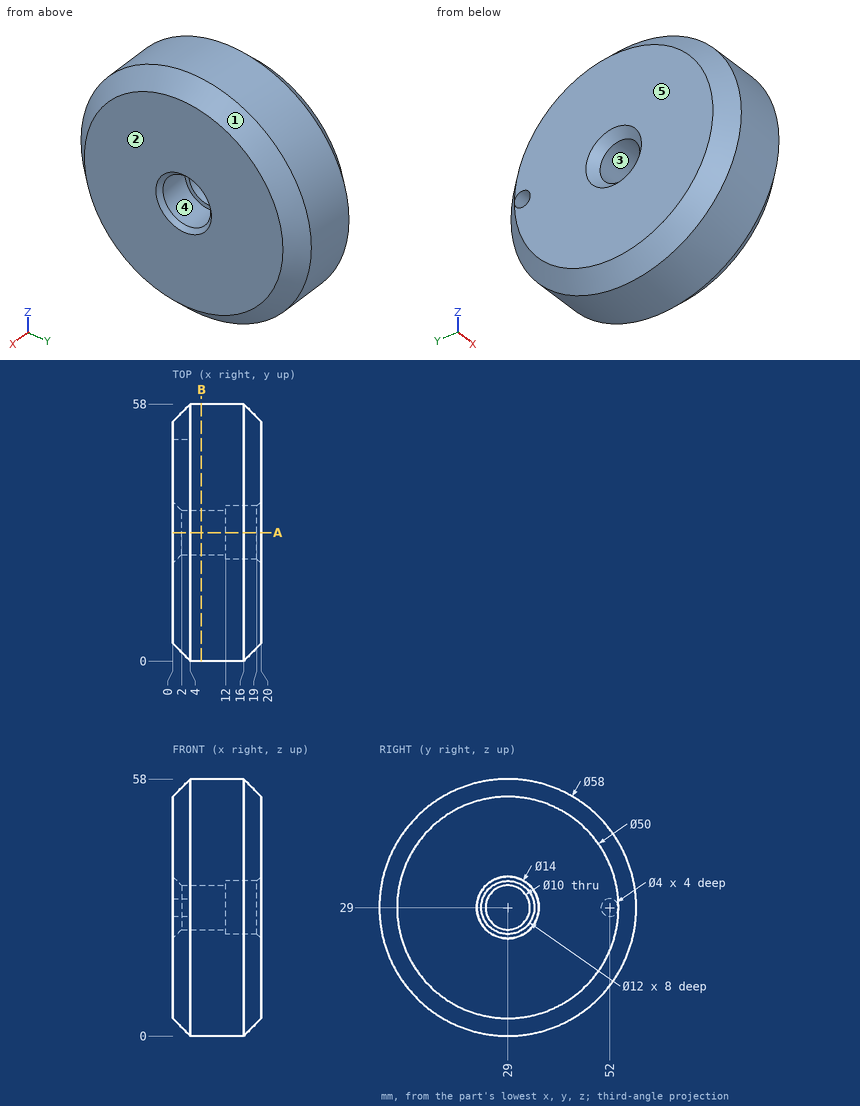
Drawing for the job (mm, zero at the part's lowest x, y, z). A direction names the side the tool comes from. Round coordinates to 2 decimals unless told otherwise and drop trailing zeros. Order: outer loops, then holes, each group sorted by start corner. A loop starts at its lowest first (then second) coordinate and runs counter-clockwise, first axis right, second up. Notation, with made-up numbers: (0, 12.25) -> (59, 12.25) arc R22 ccw to (59, 48.25) -> close; hole circle Ø10 at (-2.5, -12.75). An arc over 180 degrees is marked (long way). Write item = value, one per line. Start each with the question number.
(1) Pin check, flat tips, straight feed: P1, Ø2, axis at x = 9.5, z = 18, coming from the +Y side; P2, Ø8, axis at x = 14, y = 16.5, coming from the +Z side; P3, Ø1.5, axis at x = 12.5, z = 8.5, coming from the +Y side. Stop position of each tip, or through.
(2) Cut at A-A, the plane y = 29. List the corners of the cut face in (x, z).
(3) Probe line 1 (Z direction, x = 14.5, y = 29); line 2 (Z direction, x = 6, y = 29); line 3 (Y direction, x = 17.75, z = 29). List the from-to ranges inside material, lowest first. Write a range as [from, to].
(4) Pull direction Y, two halves, no side cores. Call the marked faces 1, 2 and 3: released by +Y, released by -Y, zero draft, split by the parting line, or undercut.
(5) Cut at B-B, the plane x = 6.5. List the corners of the cut face in (y, z).
(6) Which spindle directions (+Z, -Z, +X, -X, +Y, -Y) get a long thin tool onto all of the face, cutting with end or side? Do the marked faces 4 and 5. Say none if no direction does.
Model answer:
q1.P1 = 56.22
q1.P2 = 56.73
q1.P3 = 50.24
q2.outline = (0, 4) -> (4, 0) -> (16, 0) -> (20, 4) -> (20, 22) -> (19, 23) -> (12, 23) -> (12, 24) -> (2, 24) -> (0, 22) -> close; (0, 36) -> (2, 34) -> (12, 34) -> (12, 35) -> (19, 35) -> (20, 36) -> (20, 54) -> (16, 58) -> (4, 58) -> (0, 54) -> close
q3.line_1 = [0, 23], [35, 58]
q3.line_2 = [0, 24], [34, 58]
q3.line_3 = [1.75, 23], [35, 56.25]
q4.face_1 = split by the parting line
q4.face_2 = zero draft
q4.face_3 = undercut
q5.outline = circle Ø58 at (29, 29); hole circle Ø10 at (29, 29)
q6.face_4 = +X
q6.face_5 = +Z, -Z, -X, +Y, -Y
